The drawing under review shows one solid part. Ordinate dimensions are in mm from its lowest x, y, z. A direction names the side the tool comes from. Give positions to 0.01 mm unless a question says otherwise; leave off trailing zeros. Order: outer loops, then holes, each group sorted by start corner. A loop starts at its lowest first (then second) coordinate and runs counter-clockwise, first axis right, second up. Notation, with made-up numbers: (67, 29) -> (99, 29) arc R22 ccw to (99, 52) -> close; hole circle Ø8 at (21, 75). An arc over 180 degrees is marked (long way). One line per item, written item: value.
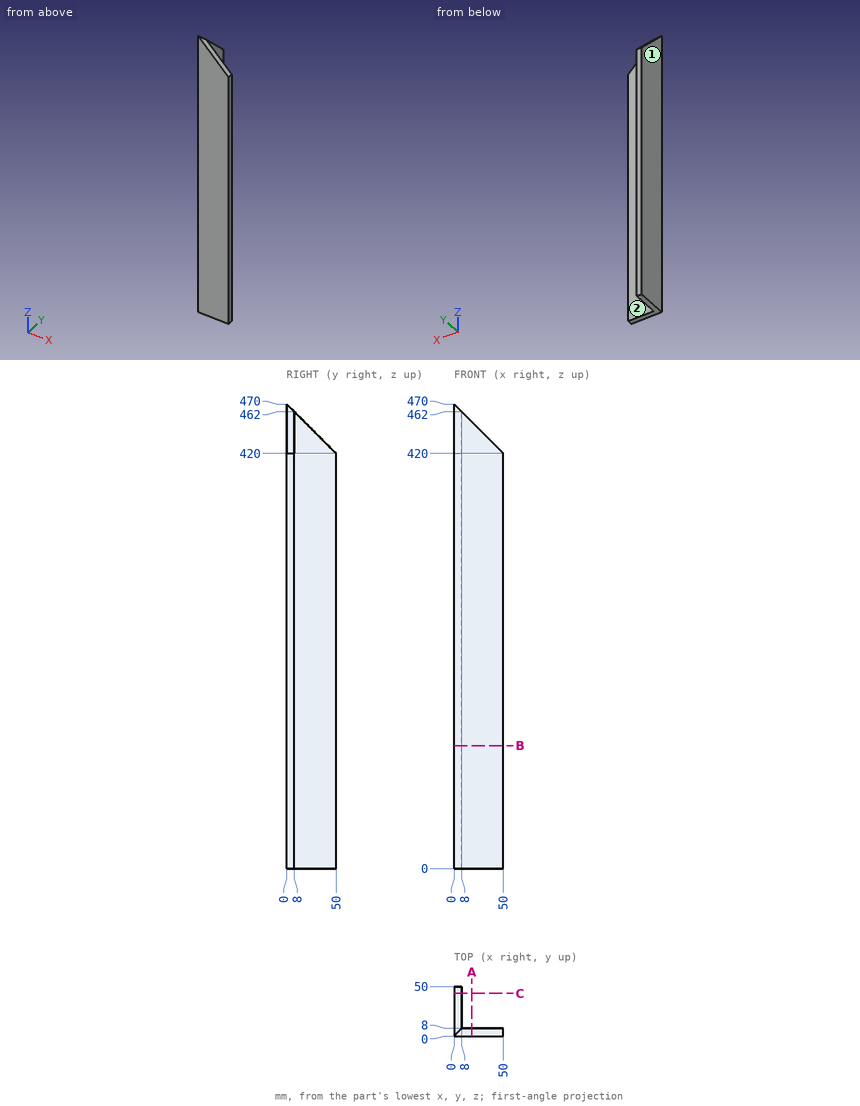
Item 1: Machinability: for the marked faces 1 and 2, which of the approach directions +Z, -Z, +X, -X, +Y, -Y give a long, thin tool a straight path to every point of the face, cutting with its end or side? Answer none if there is none.
Returned:
face 1: +Z, -Z, -X, +Y, -Y
face 2: +Z, -Z, +X, +Y
Item 2: Clearance check with flat-ended pins moving along their axes: P1, Ø12, axis at y = 35, z = 211.5, coming from the -X side; P2, Ø3, axis at y = 20.5, z = 204, coming from the +X side; P3, Ø12, axis at x = 35.5, z = 374, coming from the +Y side; P4, Ø6, axis at x = 9, y = 33.5, coming from the +Z side. State where each tip first meets the part, or that it passes through.
Returned:
P1: x = 0
P2: x = 8
P3: y = 8
P4: z = 439.33
Item 3: Add section B-B on z = 124.5. Give the boundary of the cut face in (x, y).
Returned:
outline: (0, 0) -> (50, 0) -> (50, 8) -> (8, 8) -> (8, 50) -> (0, 50) -> close
Item 4: To check wall thickness, follow line 1 along X through (y, z) = (37.5, 297.5); line 2 along Z through (x, y) = (3, 30.5). State the ranges of each line that lie inside material, in increasing order. Write a range as from..to.
Returned:
line 1: 0..8
line 2: 0..439.5
Item 5: Add section A-A on x = 18. Give the boundary of the cut face in (y, z), plus the area to 3 significant figures.
Returned:
outline: (0, 0) -> (8, 0) -> (8, 452) -> (0, 452) -> close
area: 3,620 mm²
Item 6: Add section C-C on y = 43. Give the boundary of the cut face in (x, z), plus the area to 3 significant figures.
Returned:
outline: (0, 0) -> (8, 0) -> (8, 427) -> (0, 427) -> close
area: 3,420 mm²
